CAD build for the part. Positions are in the model's coordinates, mm. A direction names the side the tool comes from. Coordinates: 2 decimals unless noted, no trailing zeros. Loops run counter-clockwise (first coordinate to the right, second up) from the corner with the lowest first, then second, coordinate; pieces in that order, holes last. Notation, with made-up numbers: (86, 4.5) -> (107, 4.5) arc R26 ccw to (107, 37.5) -> close; hole circle Ø7 at (53.25, -10.75). An arc over 180 degrees is marked (long way). Return JSON: item names as keys, results as strings. Group by question number.
(1) Saw through at A-A on y = -12.5. Write the cut outline in (x, z), then the cut area to 3 significant figures.
(2) Mould opens along Y. For faces 1 (the face through (6, -45.237, -9)), 2 (the face through (6, -1, -4)), 3 (the face through (34, -1.737, 29)), 4 (the face through (6.99, -44.73, -47.15)) say: pulls with the +Y half, pulls with the -Y half, needs draft (parallel to the pull), parting line crosses it, or undercut.
(3) Flat gauge pins, fed straight in: pin 1 Ø1.1 at (y, z) = (-45, 33.5) entering from +X; pin 2 Ø1.5 at (x, y) = (14, -17) entering from +Z; pin 3 Ø8 at (y, z) = (-19, -7) entering from +X. Where does each tip first touch, or does it go through?
(4) Tool access for faces 5 (the face through (6, -44.237, -9)), 6 (the face through (-11.737, -23, -12)), 7 (the face through (-10.737, -23, -13)): list every direction of +Z, -Z, +X, -X, +Y, -Y with a clear straight run to the whole face (end or side of a thin tool).
(5) Probe L1, parallel to X at y = -0.25, z = -40; L2, parallel to Y at x = 2, z = -5.5; L3, parallel to X at y = -3, z = -2.5. List the from-to ranges inside material, lowest first.
```python
from build123d import *

# Parameters (mm, degrees)
SM_BASE_FLANGE_1_DEPTH      = 1
SM_EDGE_FLANGE_1_DEPTH      = 60
SM_EDGE_FLANGE_2_DEPTH      = 60
SM_START                    = 1
SM_EDGE_FLANGE_2_FLAT_DEPTH = 1
SKETCH_16_R                 = 1.5
CUT_EXTRUDE_1_DEPTH         = 75.818592891
FILLET_1_R                  = 10
SM_EDGE_FLANGE_4_DEPTH      = 41.7634
SM_EDGE_FLANGE_5_DEPTH      = 41.7634


# Sheet-metal steps are written as plain solids
with BuildPart() as part:
    # Sketch 1 → 基材-凸緣1 (new body)
    with BuildSketch(Plane(origin=(0, 0, 0), x_dir=(1, 0, 0), z_dir=(0, 1, 0))):
        Polygon((-10, 0), (32.426406871, -42.426406871), (32.426406871, -14.142135624), (10, 8.284271247), (10, 50), (-10, 50), align=None)
    extrude(amount=-SM_BASE_FLANGE_1_DEPTH)

    # 邊線-凸緣1 section (across the edge) → 邊線-凸緣1 (add)
    with BuildSketch(Plane(origin=(31.905552016, -1, 42.947261726), x_dir=(0.7071067811865475, -3.4914813388431334e-15, -0.7071067811865476), z_dir=(-0.7071067811865476, 0, -0.7071067811865475))):
        with BuildLine():
            Line((-1, 0.7366), (-1, 42.5))
            Line((-1, 42.5), (0, 42.5))
            Line((0, 42.5), (0, 0.7366))
            ThreePointArc((0, 0.7366), (0.215745145, 0.215745145), (0.7366, 0))
            Line((0.7366, 0), (0.7366, -1))
            ThreePointArc((0.7366, -1), (-0.491361636, -0.491361636), (-1, 0.7366))
        make_face()
    extrude(amount=SM_EDGE_FLANGE_1_DEPTH)

    # 邊線-凸緣2 bend section (across the edge) → 邊線-凸緣2 (add)
    with BuildSketch(Plane(origin=(31.905552016, -44.2366, 42.947261726), x_dir=(0, 1, 0), z_dir=(-0.7071067811865477, 0, -0.7071067811865475))):
        with BuildLine():
            Line((-1, 0.7366), (0, 0.7366))
            ThreePointArc((0, 0.7366), (0.215745145, 0.215745145), (0.7366, 0))
            Line((0.7366, 0), (0.7366, -1))
            ThreePointArc((0.7366, -1), (-0.491361636, -0.491361636), (-1, 0.7366))
        make_face()
    extrude(amount=SM_EDGE_FLANGE_2_DEPTH)

    # 邊線-凸緣2 profile (on flange) → 邊線-凸緣2 flat (add)
    with BuildSketch(Plane(origin=(-5.520854855, -44.2366, 5.520854855), x_dir=(-0.7071067811865477, 0, -0.7071067811865475), z_dir=(0, -1, 0)).offset(SM_START)):
        Polygon((7.071067812, 0.7366), (42.426406871, 36.091939059), (28.284271247, 50.234074683), (-1.213203436, 20.7366), (-32.928932188, 20.7366), (-52.928932188, 0.7366), align=None)
    extrude(amount=-SM_EDGE_FLANGE_2_FLAT_DEPTH)

    # 草圖16 → 除料-伸長1 (cut, through all)
    with BuildSketch(Plane(origin=(0, 0, 0), x_dir=(1, 0, 0), z_dir=(0, 1, 0))):
        with Locations(Location((0, 40, 0), (0, 0, 270))):
            Circle(SKETCH_16_R)
        with BuildLine():
            ThreePointArc((3.428571429, 47.228063223), (0, 48), (-3.428571429, 47.228063223))
            ThreePointArc((-3.428571429, 47.228063223), (-3.903507903, 45.895983892), (-2.571428571, 45.421047417))
            ThreePointArc((-2.571428571, 45.421047417), (0, 46), (2.571428571, 45.421047417))
            ThreePointArc((2.571428571, 45.421047417), (3.903507903, 45.895983892), (3.428571429, 47.228063223))
        make_face()
        with BuildLine():
            ThreePointArc((7.228063223, 36.571428571), (8, 40), (7.228063223, 43.428571429))
            ThreePointArc((7.228063223, 43.428571429), (5.895983892, 43.903507903), (5.421047417, 42.571428571))
            ThreePointArc((5.421047417, 42.571428571), (6, 40), (5.421047417, 37.428571429))
            ThreePointArc((5.421047417, 37.428571429), (5.895983892, 36.096492097), (7.228063223, 36.571428571))
        make_face()
        with BuildLine():
            ThreePointArc((-3.428571429, 32.771936777), (0, 32), (3.428571429, 32.771936777))
            ThreePointArc((3.428571429, 32.771936777), (3.903507903, 34.104016108), (2.571428571, 34.578952583))
            ThreePointArc((2.571428571, 34.578952583), (0, 34), (-2.571428571, 34.578952583))
            ThreePointArc((-2.571428571, 34.578952583), (-3.903507903, 34.104016108), (-3.428571429, 32.771936777))
        make_face()
        with BuildLine():
            ThreePointArc((-7.228063223, 43.428571429), (-8, 40), (-7.228063223, 36.571428571))
            ThreePointArc((-7.228063223, 36.571428571), (-5.895983892, 36.096492097), (-5.421047417, 37.428571429))
            ThreePointArc((-5.421047417, 37.428571429), (-6, 40), (-5.421047417, 42.571428571))
            ThreePointArc((-5.421047417, 42.571428571), (-5.895983892, 43.903507903), (-7.228063223, 43.428571429))
        make_face()
    extrude(amount=-CUT_EXTRUDE_1_DEPTH, mode=Mode.SUBTRACT)

    # 圓角1
    fillet_1_edges = [part.edges().sort_by_distance(p)[0] for p in [
        (-10, -0.5, -50),
        (10, -0.5, -50),
        (-10, -44.7366, -50),
        (10, -44.7366, -50),
    ]]
    fillet(fillet_1_edges, radius=FILLET_1_R - 0.0001)  # a hair under: the kernel refuses the full size

    # 邊線-凸緣4 section (across the edge) → 邊線-凸緣4 (add)
    with BuildSketch(Plane(origin=(33.163006871, -1.7366, 44.204716581), x_dir=(-1, 0, 0), z_dir=(0, -1, 0))):
        with BuildLine():
            Line((-1, 1.77830971), (-1, 30.062580958))
            Line((-1, 30.062580958), (0, 30.062580958))
            Line((0, 30.062580958), (0, 1.77830971))
            ThreePointArc((0, 1.77830971), (0.454715384, 1.097780046), (1.257454855, 1.257454855))
            Line((1.257454855, 1.257454855), (1.964561636, 0.550348074))
            ThreePointArc((1.964561636, 0.550348074), (0.072031951, 0.173900514), (-1, 1.77830971))
        make_face()
    extrude(amount=SM_EDGE_FLANGE_4_DEPTH)

    # 邊線-凸緣5 section (across the edge) → 邊線-凸緣5 (add)
    with BuildSketch(Plane(origin=(-10.7366, -43.5, 0.30510971), x_dir=(1, 0, 0), z_dir=(0, 1, 0))):
        with BuildLine():
            Line((-1, 0.30510971), (-1, 25))
            Line((-1, 25), (0, 25))
            Line((0, 25), (0, 0.30510971))
            ThreePointArc((0, 0.30510971), (0.056070336, 0.023225094), (0.215745145, -0.215745145))
            Line((0.215745145, -0.215745145), (-0.491361636, -0.922851926))
            ThreePointArc((-0.491361636, -0.922851926), (-0.867809196, -0.359458339), (-1, 0.30510971))
        make_face()
    extrude(amount=SM_EDGE_FLANGE_5_DEPTH)


solid = part.part
```
Geometry results:
{
 "1": {"outline": "(-11.74, -24.69) -> (-10.74, -24.69) -> (-10.74, 0) arc R0.74 cw to (-10.52, 0.52) -> (31.91, 42.95) arc R0.74 cw to (33.16, 42.43) -> (33.16, 14.14) -> (34.16, 14.14) -> (34.16, 42.43) arc R1.74 ccw to (31.2, 43.65) -> (-11.23, 1.23) arc R1.74 ccw to (-11.74, 0) -> close", "area": "117 mm²"},
 "2": {"face 1": "pulls with the -Y half", "face 2": "undercut", "face 3": "pulls with the +Y half", "face 4": "needs draft"},
 "3": {"pin 1": "x = 32.43", "pin 2": "z = 27.21", "pin 3": "x = -10.74"},
 "4": {"face 5": "-Z, +X", "face 6": "+Z, -Z, -X, +Y, -Y", "face 7": "-Z, +X, +Y, -Y"},
 "5": {"L1": "-10 to -8, -6 to -1.5, 1.5 to 6, 8 to 10", "L2": "-45.24 to -44.24, -1 to 0", "L3": "-11.74 to -10.74"}
}
